from build123d import *

# Parameters (mm, degrees)
CHAMFER_1_SIZE = 0.2


with BuildPart() as part:
    # 草图1 → 旋转1 (revolve)
    with BuildSketch(Plane.XY, mode=Mode.PRIVATE) as revolve_1_sk:
        Polygon((0, 1.5), (0, 6.692857143), (-1, 6.692857143), (-1, 2.75), (-3, 2.75), (-3, 1.5), align=None)
    revolve(revolve_1_sk.sketch.rotate(Axis((-9.1, 0, 0), (1, 0, 0)), 90), axis=Axis((-9.1, 0, 0), (1, 0, 0)))

    # 倒角1
    chamfer_1_edges = [part.edges().sort_by_distance(p)[0] for p in [
        (-3, 0, -1.5),
        (-3, 0, -2.75),
    ]]
    chamfer(chamfer_1_edges, length=CHAMFER_1_SIZE)


solid = part.part
Work out the finished part from the listing and answer in its coordinate system (mm). A direction names the side the tool comes from. Give positions to 0.01 mm unless a question says otherwise; leave off trailing zeros. Write each loop counter-clockwise with the first axis right and the second up, starting at its lowest first coordinate (ties: lowest second). Pieces come first, ordered by that corner, then holes. Notation, with made-up numbers: M -31.75,-21.75 L -9.75,-21.75 A13 ccw -9.75,-4.75 Z; hole C 71,45 d3. An arc over 180 degrees is marked long. Answer as CSV lines item,"result".
Q1. Given P1, Ø1.5, axis at x = -1.5, z = -4.5, coming from the -Y side, flat-ended and moving along its own axis, determine where the tip first touches the part or whether it passes through.
A:
P1,"stops at y = -5.41"
Q2. A tool of negligible diameter and unlimited length cuts with its end or side. For faces 4 (the flat face through (-1, 3, 0)), 5 (the flat face through (0, -2, 0)), from which of +Z, -Z, +X, -X, +Y, -Y can it reach the whole face along a straight path? Write none if from no direction.
A:
face 4,"-X"
face 5,"+Z, -Z, +X, +Y, -Y"
Q3. Find the intervals of material crossed by probe 1 along Y at (x, z) = (-0.7, 0); probe 2 along Y at (x, z) = (-2.05, 0); probe 3 along X at (y, z) = (1, -2.75), in increasing order. Write a range as [from, to].
A:
probe 1,"y = [-6.69, -1.5], [1.5, 6.69]"
probe 2,"y = [-2.75, -1.5], [1.5, 2.75]"
probe 3,"x = [-1, 0]"
Q4. A cutting plane is placed at A-A on y = 0. Write down the section's boundary in (x, z), plus the area to 3 significant figures.
A:
outline,"M -3,-2.55 L -2.8,-2.75 L -1,-2.75 L -1,-6.69 L 0,-6.69 L 0,-1.5 L -2.8,-1.5 L -3,-1.7 Z; M -3,1.7 L -2.8,1.5 L 0,1.5 L 0,6.69 L -1,6.69 L -1,2.75 L -2.8,2.75 L -3,2.55 Z"
area,"15.3 mm²"
Q5. A cutting plane is placed at C-C on x = -0.3. Write down the section's boundary in (y, z), plus the area to 3 significant figures.
A:
outline,"C 0,0 d13.39; hole C 0,0 d3"
area,"134 mm²"
Q6. The mould has two halves that part along Z. Classify faces 1 (the flat face through (-3, 1, 2)), 2 (the cylindrical face through (-0.507, -6.636, -0.871)), 3 (the cylindrical face through (-1.38, -0.45, 1.43)): +Z half, -Z half, draft (parallel to the pull), parting line (faces both ways), or undercut.
A:
face 1,"draft"
face 2,"parting line"
face 3,"undercut"
Q7. A cutting plane is placed at D-D on y = 5. Write down the section's boundary in (x, z), plus the area to 3 significant figures.
A:
outline,"M -1,-4.45 L 0,-4.45 L 0,4.45 L -1,4.45 Z"
area,"8.90 mm²"
